from build123d import *

# Parameters (mm, degrees)
F1_W         = 17.78
F1_H         = 30.48
F2_DEPTH     = 5.08
F3_W         = 17.78
F3_H         = 5.08
F4_DEPTH     = 38.1
F6_W         = 17.78
F6_H         = 5.08
F7_DEPTH     = 25.4
F9_W         = 17.78
F9_H         = 5.08
F10_DEPTH    = 7.62
F11_R        = 1.27
F12_R        = 1.27
F13_T1_DEPTH = 41.91
F13_T3_DEPTH = 30.48
F16_DEPTH    = 1.905


# Not quite as in the source:
# - a fillet or chamfer that OpenCascade refuses, or shapes differently, is made with other operations: its cross-section is extruded or revolved along the edge and cut away or added


with BuildPart() as f2:
    # F1 (on offset) → F2 (new body)
    with BuildSketch(Plane.XY.offset(25.4)):
        with Locations((-1.3240431021, 15.24)):
            Rectangle(F1_W, F1_H)
    extrude(amount=F2_DEPTH)

    # F3 (on offset) → F4 (join)
    with BuildSketch(Plane.XY.offset(25.4)):
        with Locations((-1.1914440245, 2.54)):
            Rectangle(F3_W, F3_H)
    extrude(amount=-F4_DEPTH)

    # F6 (on offset) → F7 (join)
    with BuildSketch(Plane(origin=(0, 5.08, 0), x_dir=(-1, 0, 0), z_dir=(0, 1, 0))):
        with Locations((1.1914440245, -10.16)):
            Rectangle(F6_W, F6_H)
    extrude(amount=F7_DEPTH)

    # F9 (on offset) → F10 (join)
    with BuildSketch(Plane.XY.offset(-7.62)):
        with Locations((-1.1914440245, 27.94)):
            Rectangle(F9_W, F9_H)
    extrude(amount=F10_DEPTH)

    # F11
    f11_edges = [f2.edges().sort_by_distance(p)[0] for p in [
        (-1.191444, 30.48, 0),
        (-10.081444, 27.94, 0),
        (-1.191444, 25.4, 0),
        (7.698556, 27.94, 0),
        (-1.191444, 30.48, -12.7),
        (-10.081444, 30.48, -6.35),
        (7.698556, 30.48, -6.35),
    ]]
    fillet(f11_edges, radius=F11_R)

    # F12
    f12_edges = [f2.edges().sort_by_distance(p)[0] for p in [
        (7.565957, 30.48, 27.94),
        (-10.214043, 30.48, 27.94),
        (-1.324043, 30.48, 25.4),
        (-1.324043, 30.48, 30.48),
    ]]
    fillet(f12_edges, radius=F12_R)

    # F13: fillet of radius 2.54 on 4 edges, made by hand

    # F13_s2 → F13_t1 (cut)
    with BuildSketch(Plane.XZ.offset(-35.56)):
        with BuildLine():
            ThreePointArc((-10.2140431021, 27.94), (-9.4700943263, 29.7360512242), (-7.6740431021, 30.48))
            Line((-7.6740431021, 30.48), (-10.2140431021, 30.48))
            Line((-10.2140431021, 30.48), (-10.2140431021, 27.94))
        make_face()
        with BuildLine():
            ThreePointArc((7.5659568979, 27.94), (6.8220081221, 29.7360512242), (5.0259568979, 30.48))
            Line((5.0259568979, 30.48), (7.5659568979, 30.48))
            Line((7.5659568979, 30.48), (7.5659568979, 27.94))
        make_face()
    extrude(amount=F13_T1_DEPTH, mode=Mode.SUBTRACT)

    # F13_s4 → F13_t3 (cut)
    with BuildSketch(Plane.YZ.offset(-16.5640431021)):
        with BuildLine():
            ThreePointArc((0, 27.94), (0.7439487758, 29.7360512242), (2.54, 30.48))
            Line((2.54, 30.48), (0, 30.48))
            Line((0, 30.48), (0, 27.94))
        make_face()
    extrude(amount=F13_T3_DEPTH, mode=Mode.SUBTRACT)

    # F15 (on offset) → F16 (join, symmetric)
    with BuildSketch(Plane.YZ.offset(-1.1914440245)):
        Polygon((-20.4633865505, 4.2401612736), (0, 4.2401612736), (0, 8.0501612736), (-16.6533865505, 8.0501612736), (-16.6533865505, 14.932741411), (-20.4633865505, 14.932741411), align=None)
    extrude(amount=F16_DEPTH, both=True)


solid = f2.part
The model under review builds one solid part; all positions refer to its coordinate system, in mm. A direction names the side the tool comes from. Coordinates: 2 decimals unless noted, no trailing zeros. Loops run counter-clockwise (first coordinate to the right, second up) from the corner with the lowest first, then second, coordinate; pieces in that order, holes last.
(1) Draft analysis for pull direction Y (two halves, no side actions). For faces 4 (the flat face through (-1, 5.08, 9)), 5 (the flat face through (0.714, -13, 7)), 6 (the cylindrical face through (-1.2, 30.098, 25.762)), 7 (the flat face through (-1, -16.653, 11)), state which applies: +Y half, -Y half, draft (parallel to the pull), parting line (faces both ways), or undercut.
Determined:
face 4: undercut
face 5: draft
face 6: +Y half
face 7: undercut
(2) Insertion check: P1, Ø5.5, axis at y = -9.5, z = 9.5, coming from the +X side; P2, Ø3, axis at x = -0.5, y = -11, coming from the -Z side; P3, Ø8.5, axis at y = -13, z = 11.5, coming from the -X side; P4, Ø6, axis at y = 10, z = 20, coming from the +X side. Each pin has a flat end and moves straight along its axis. Give the tip position at first contact, or say it passes through.
Determined:
P1: stops at x = 0.71
P2: stops at z = 4.24
P3: stops at x = -3.1
P4: passes through
(3) Consider section A-A, the plane y = 16.5. Give the boundary of the cut face in (x, z), plus the area to 3 significant figures.
Determined:
outline: (-10.21, 25.4) - (7.57, 25.4) - (7.57, 27.94) arc R2.54 ccw to (5.03, 30.48) - (-7.67, 30.48) arc R2.54 ccw to (-10.21, 27.94) - close; (-10.08, -12.7) - (7.7, -12.7) - (7.7, -7.62) - (-10.08, -7.62) - close
area: 178 mm2
(4) Consider section D-D, the plane z = 11. Give the boundary of the cut face in (x, y).
Determined:
outline: (-10.08, 0) - (7.7, 0) - (7.7, 5.08) - (-10.08, 5.08) - close; (-3.1, -20.46) - (0.71, -20.46) - (0.71, -16.65) - (-3.1, -16.65) - close
(5) Wall thickness on L1, parallel to Z at x = 4, y = 25; L2, parallel to Y at x = 0.25, z = -6; L3, parallel to X at y = 1.5, z = -8.5: over which ranges is each line inside the solid? List them lowest first.
Determined:
L1: z = -12.7 to -7.62, 25.4 to 30.48
L2: y = 0 to 5.08, 25.4 to 30.48
L3: x = -10.08 to 7.7
(6) Consider section B-B, the plane z = -6.5. Give the boundary of the cut face in (x, y).
Determined:
outline: (-10.08, 0) - (7.7, 0) - (7.7, 5.08) - (-10.08, 5.08) - close; (-10.08, 25.4) - (7.7, 25.4) - (7.7, 29.21) arc R1.27 ccw to (6.43, 30.48) - (-8.81, 30.48) arc R1.27 ccw to (-10.08, 29.21) - close
(7) Consider section C-C, the plane x = 4. Give the boundary of the cut face in (y, z).
Determined:
outline: (0, -12.7) - (29.21, -12.7) arc R1.27 ccw to (30.48, -11.43) - (30.48, -1.27) arc R1.27 ccw to (29.21, 0) - (26.67, 0) arc R1.27 ccw to (25.4, -1.27) - (25.4, -7.62) - (5.08, -7.62) - (5.08, 25.4) - (29.21, 25.4) arc R1.27 ccw to (30.48, 26.67) - (30.48, 29.21) arc R1.27 ccw to (29.21, 30.48) - (2.54, 30.48) arc R2.54 ccw to (0, 27.94) - close
(8) Tool access review of faces 1 (the cylindrical face through (-1.067, 25.782, -0.362)), 2 (the flat face through (-1, -19, 14.933)), 3 (the flat face through (-3.096, -13, 7)): name each direction out of +Z, -Z, +X, -X, +Y, -Y from which nothing blocks a thin tool from reaching the whole face with its end or side.
Determined:
face 1: +X, -X
face 2: +Z, +X, -X, -Y
face 3: +Z, -Z, -X, -Y
